from build123d import *

# Parameters (mm, degrees)
F0_W     = 66.2185922265
F0_H     = 111.7807626724
F1_DEPTH = 10.16
F2_R     = 2.032
F3_T     = -4.064


# Not quite as in the source:
# - two fillets or chamfers of one size are made in one step


with BuildPart() as f1:
    # F0 (on Front) → F1 (new body)
    with BuildSketch(Plane.XZ):
        with Locations((-33.1092961133, 55.8903813362)):
            Rectangle(F0_W, F0_H)
    extrude(amount=F1_DEPTH)

    # F2
    f2_edges = [f1.edges().sort_by_distance(p)[0] for p in [
        (0, -10.16, 55.890381),
        (-66.218592, -10.16, 55.890381),
        (0, -5.08, 111.780763),
        (-66.218592, -5.08, 111.780763),
        (-33.109296, -10.16, 111.780763),
    ]]
    fillet(f2_edges, radius=F2_R)

    # F3
    f3_openings = [f1.faces().sort_by_distance(p)[0] for p in [
        (-33.109296, 0, 55.877105),
    ]]
    offset(amount=F3_T, openings=f3_openings)


solid = f1.part
Design review of the part built by this model. Coordinates are the model's own, in mm. A direction names the side the tool comes from. Coordinates: 2 decimals unless noted, no trailing zeros. Loops run counter-clockwise (first coordinate to the right, second up) from the corner with the lowest first, then second, coordinate; pieces in that order, holes last. Notation, with made-up numbers: M -11.75,52 L 36.25,52 A31 cw 36.25,77 Z; hole C -30,49.25 d7. An arc over 180 degrees is marked long. Answer as CSV lines item,"result".
Item 1: For P1, Ø17.5, axis at x = -23.5, z = 80, coming from the +Y side, flat-tipped, find the tip position at first contact; note if it passes through.
Answer list:
P1,"y = -6.1"
Item 2: Machinability: for faces 5 (the face through (-62.155, -3, 55)), 6 (the face through (-63, 0, 60)), which of the approach directions +Z, -Z, +X, -X, +Y, -Y give a long, thin tool a straight path to every point of the face, cutting with its end or side? Answer none if there is none.
Answer list:
face 5,"+Y"
face 6,"+Z, -Z, +X, -X, +Y"
Item 3: For probe 1 along X at (y, z) = (-5.5, 45.5); probe 2 along Z at (x, y) = (-20.5, -1.25); probe 3 along Y at (x, z) = (-12.5, 53), list the stretches that pass through material, from the lowest coordinate up.
Answer list:
probe 1,"-66.22 to -62.15, -4.06 to 0"
probe 2,"0 to 4.06, 107.72 to 111.78"
probe 3,"-10.16 to -6.1"
Item 4: Add section C-C on x = -21.5. State the section outline as (y, z) points, plus the area to 3 significant figures.
Answer list:
outline,"M -10.16,0 L 0,0 L 0,4.06 L -6.1,4.06 L -6.1,107.72 L 0,107.72 L 0,111.78 L -8.13,111.78 A2.03 ccw -10.16,109.75 Z"
area,"503 mm²"
Item 5: Add section A-A on z = 14.5. State the section outline as (x, y) points, plus the area to 3 significant figures.
Answer list:
outline,"M -66.22,-8.13 A2.03 ccw -64.19,-10.16 L -2.03,-10.16 A2.03 ccw 0,-8.13 L 0,0 L -4.06,0 L -4.06,-6.1 L -62.15,-6.1 L -62.15,0 L -66.22,0 Z"
area,"317 mm²"
Item 6: The part is to be moulded in two halves that separate along X. For faces 1 (the face through (-34, -6.096, 57)), 2 (the face through (-4.064, -3, 55)), 3 (the face through (-66.219, -4, 54)), 4 (the face through (-0.58, -9.55, 55.64)), say which applies: pulls with the +X half, pulls with the -X half, needs draft (parallel to the pull), parting line crosses it, or undercut.
Answer list:
face 1,"undercut"
face 2,"undercut"
face 3,"pulls with the -X half"
face 4,"pulls with the +X half"
Item 7: Add section B-B on y = -3.75. State the section outline as (x, z) points, plus the area to 3 significant figures.
Answer list:
outline,"M -66.22,0 L 0,0 L 0,109.75 A2.03 ccw -2.03,111.78 L -64.19,111.78 A2.03 ccw -66.22,109.75 Z; hole M -62.15,4.06 L -4.06,4.06 L -4.06,107.72 L -62.15,107.72 Z"
area,"1,380 mm²"
